Input: part model. Units: mm. Frame: model coordinates. Face numbers are marked on the shaded views. A direction names the side the tool comes from. Coordinates: 2 decimals unless noted, no trailing zeros. Loops run counter-clockwise (first coordinate to the right, second up) from the corner with the lowest first, then second, coordinate; pieces in that order, holes last. Notation, with made-up numbers: (7.5, 41) -> (54.5, 41) arc R36 cw to (54.5, 80) -> close; hole circle Ø9 at (79.5, 12.5). An arc over 180 degrees is marked (long way). Put each result on its own line as item: value. Start each with the question number.
1) Pull-direction query (X, two-part tool) for the marked faces 1, 2, 3 and 4; classes: pulls with the +X half, pulls with the -X half, needs draft (parallel to the pull), parting line crosses it, or undercut.
2) Cut plane B-B (z = 13). Return the cut outline in (x, y), plus the area to 3 significant figures.
3) Contact query for flat-ended pins moving along their axis: P1, Ø8, axis at x = 8, z = 9, coming from the -Y side; P2, Ø5, axis at x = 0, z = 13, coming from the +Y side. Output: stop coordinate, or through.
4) Material intervals for L1, parallel to X at y = 2.1, z = 13; L2, parallel to Y at x = 0.5, z = 3.25; L3, parallel to Z at x = 2, y = 2.5, sorted ascending.
5) Cut plane D-D (x = -10). Return the cut outline in (y, z).
6) Cut plane C-C (y = -2.5). Return the cut outline in (x, z).
7) Cut plane A-A (x = 0). Return the cut outline in (y, z).
8) Set-up query: the marked faces 5 and 6. Return all of +Z, -Z, +X, -X, +Y, -Y with unobstructed straight access to the full face (end or side cutting, diameter ignored); none if empty.
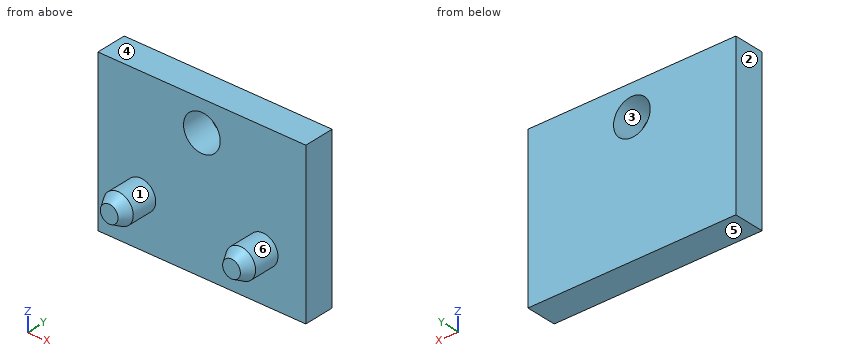
from build123d import *

# Parameters (mm, degrees)
SKETCH1_R             = 2.45
BOSS_EXTRUDE1_DEPTH   = 6
BOSS_EXTRUDE1_2_DEPTH = 6
CHAMFER1_SIZE         = 1
CHAMFER1_SIZE2        = 1.732050808
CHAMFER2_SIZE         = 1
CHAMFER2_SIZE2        = 1.732050808
SKETCH3_W             = 34
SKETCH3_H             = 26
BOSS_EXTRUDE2_DEPTH   = 5
SKETCH6_R             = 3
CUT_EXTRUDE2_DEPTH    = 26.475478406


with BuildPart() as part:
    # Sketch1 → Boss-Extrude1 (new body)
    with BuildSketch(Plane(origin=(0, 0, 0), x_dir=(1, 0, 0), z_dir=(0, 1, 0))):
        with Locations(Location((-10, 0, 0), (0, 0, 270))):
            Circle(SKETCH1_R)
    extrude(amount=-BOSS_EXTRUDE1_DEPTH)

    # Chamfer2
    chamfer2_edges = [part.edges().sort_by_distance(p)[0] for p in [
        (-10, -6, -2.45),
    ]]
    chamfer2_side = [part.faces().sort_by_distance(p)[0] for p in [
        (-10, -6, 0),
    ]]
    chamfer(chamfer2_edges, length=CHAMFER2_SIZE, length2=CHAMFER2_SIZE2, reference=chamfer2_side[0])



with BuildPart() as body_2:
    # Sketch1 → Boss-Extrude1 2 (new body)
    with BuildSketch(Plane(origin=(0, 0, 0), x_dir=(1, 0, 0), z_dir=(0, 1, 0))):
        with Locations(Location((10, 0, 0), (0, 0, 270))):
            Circle(SKETCH1_R)
    extrude(amount=-BOSS_EXTRUDE1_2_DEPTH)

    # Chamfer1
    chamfer1_edges = [body_2.edges().sort_by_distance(p)[0] for p in [
        (10, -6, -2.45),
    ]]
    chamfer1_side = [body_2.faces().sort_by_distance(p)[0] for p in [
        (10, -6, 0),
    ]]
    chamfer(chamfer1_edges, length=CHAMFER1_SIZE, length2=CHAMFER1_SIZE2, reference=chamfer1_side[0])


with BuildPart() as part_1:
    add(part.part)

    add(body_2.part)  # Boss-Extrude2 merges body 2
    # Sketch3 → Boss-Extrude2 (add)
    with BuildSketch(Plane(origin=(0, 0, 0), x_dir=(1, 0, 0), z_dir=(0, 1, 0))):
        with Locations((0, -5)):
            Rectangle(SKETCH3_W, SKETCH3_H)
    extrude(amount=BOSS_EXTRUDE2_DEPTH)

    # Sketch6 → Cut-Extrude2 (cut, through all)
    with BuildSketch(Plane.XZ):
        with Locations(Location((0, 13, 0), (0, 0, 270))):
            Circle(SKETCH6_R)
    extrude(amount=-CUT_EXTRUDE2_DEPTH, mode=Mode.SUBTRACT)


solid = part_1.part
Results found:
1. face 1: undercut
1. face 2: pulls with the -X half
1. face 3: undercut
1. face 4: needs draft
2. outline: (-17, 0) -> (-3, 0) -> (-3, 5) -> (-17, 5) -> close; (3, 0) -> (17, 0) -> (17, 5) -> (3, 5) -> close
2. area: 140 mm2
3. P1: stops at y = 0
3. P2: passes through
4. L1: x = -17 to -3, 3 to 17
4. L2: y = 0 to 5
4. L3: z = -8 to 10.76, 15.24 to 18
5. outline: (-6, -1.45) -> (-4.27, -2.45) -> (0, -2.45) -> (0, -8) -> (5, -8) -> (5, 18) -> (0, 18) -> (0, 2.45) -> (-4.27, 2.45) -> (-6, 1.45) -> close
6. outline: circle Ø4.9 at (-10, 0); circle Ø4.9 at (10, 0)
7. outline: (0, -8) -> (5, -8) -> (5, 10) -> (0, 10) -> close; (0, 16) -> (5, 16) -> (5, 18) -> (0, 18) -> close
8. face 5: -Z, +X, -X, +Y, -Y
8. face 6: -Y
